Verification items for the finished model (mm, model axes). A direction names the side the tool comes from. Give positions to 0.01 mm unless a question says otherwise; leave off trailing zeros. Order: outer loops, then holes, each group sorted by start corner. A loop starts at its lowest first (then second) coordinate and runs counter-clockwise, first axis right, second up. Notation, with made-up numbers: (32, 63.25) -> (60, 63.25) arc R27 ccw to (60, 88.25) -> close; hole circle Ø1 at (-12.5, 7). An arc over 180 degrees is marked (long way). One line per question, with ' | ' between items. Start each with the question number.
Q1. Mould release check, pull along X, two halves, no side actions. Record for faces 1 (the cylindrical face through (9, 3, 0)), 2 (the flat face through (-130, 0, 0)), 3 (the cylindrical face through (-1.82, -4.76, 3.65)): released by +X, released by -X, zero draft, split by the parting line, or undercut.
Q2. Go/stop test with flat-tipped pins: pin 1 (3.5 mm diameter, centred on x = 7, z = 0, fed in from +Y); pin 2 (3 mm diameter, centred on x = -115, z = 2.5, fed in from +Y); pin 3 (1.5 mm diameter, centred on x = -45, y = -3.5, fed in from -Z). Record where each tip stops, or that it passes through.
Q3. Section check A-A on z = 0. Record the cut outline in (x, y).
Q4. Section check B-B on y = -2.25. Record the cut outline in (x, z).
Q5. Access from +Z, -Z, +X, -X, +Y, -Y to the whole of each face (thin tool, end or side, straight path). Record for faces 4 (the flat face through (7, 0, 0)), 5 (the flat face through (130, 0, 0)), 6 (the flat face through (115, 3, 0)).
Q6. Section check C-C on x = -44. Record the cut outline in (y, z).
Q7. Material ranges on probe 1 along X at (y, z) = (1.5, 0); probe 2 along X at (y, z) = (4.5, 0); probe 3 along X at (y, z) = (4.5, 3.5), recorded low to high. Write a range as [from, to].
Autodesk Inventor part; units mm, degrees
ref_plane "YZ Plane" through (0, 0, 0) normal (1, 0, 0) x (0, 1, 0)
ref_plane "XZ Plane" through (0, 0, 0) normal (0, 1, 0) x (-1, 0, 0)
ref_plane "XY Plane" through (0, 0, 0) normal (0, 0, 1) x (1, 0, 0)
sketch "Sketch1" plane through (0, 0, 0) normal (1, 0, 0) x (0, 1, 0)
  circle A0 centre (0, 0) radius 6
  dimension "d0" = 12
extrude "Extrusion1" add sketch "Sketch1" along normal mid plane 260
sketch "Sketch2" plane through (0, 0, 0) normal (0, 0, 1) x (1, 0, 0)
  line L0 (-130, 6) -> (-130, -6)
  line L1 (-130, 0) -> (-115, 0)
  line L2 (-115, 0) -> (-115, 6)
  line L3 (130, -6) -> (130, 6)
  line L4 (130, 0) -> (115, 0)
  line L5 (115, 0) -> (115, 6)
  line L6 (112, 9) -> (118, 9)
  line L7 (118, 9) -> (118, 3)
  line L8 (118, 3) -> (112, 3)
  line L9 (112, 3) -> (112, 9)
  line L10 (112, 9) -> (118, 3) construction
  line L11 (118, 9) -> (112, 3) construction
  line L12 (-118, 9) -> (-112, 9)
  line L13 (-112, 9) -> (-112, 3)
  line L14 (-112, 3) -> (-118, 3)
  line L15 (-118, 3) -> (-118, 9)
  line L16 (-118, 9) -> (-112, 3) construction
  line L17 (-112, 9) -> (-118, 3) construction
  point P0 (0, 0)
  dimension "d3" = 15
  dimension "d4" = 15
  dimension "d5" = 6
  dimension "d6" = 6
extrude "Extrusion2" cut sketch "Sketch2" along normal mid plane 20
sketch "Sketch3" plane through (0, 0, 0) normal (0, 1, 0) x (-1, 0, 0)
  line L0 (-130, 6) -> (-130, -6)
  line L1 (-130, -6) -> (-5, -6)
  line L2 (130, -6) -> (-130, -6)
  line L3 (-5, -6) -> (-5, 0)
  line L4 (130, 6) -> (-130, 6)
  line L5 (-5, 0) -> (5, 0)
  line L6 (5, 0) -> (7, 0)
  line L7 (-5, 0) -> (-7, 0)
  circle A0 centre (7, 0) radius 2
  circle A1 centre (-7, 0) radius 2
  point P0 (0, 0)
  dimension "d9" = 125
  dimension "d10" = 10
  dimension "d11" = 2
  dimension "d12" = 2
extrude "Extrusion3" cut sketch "Sketch3" along normal blind 10
thread "Thread1"
thread "Thread2"
properties part number "base_axis_12mm" material "Stainless Steel"
Filled in:
1) face 1: undercut | face 2: released by -X | face 3: zero draft
2) pin 1: y = 0 | pin 2: y = 3 | pin 3: z = -5.33
3) outline: (-130, -6) -> (130, -6) -> (130, 6) -> (118, 6) -> (118, 3) -> (112, 3) -> (112, 6) -> (9, 6) -> (9, 0) -> (5, 0) -> (5, 6) -> (-5, 6) -> (-5, 0) -> (-9, 0) -> (-9, 6) -> (-112, 6) -> (-112, 3) -> (-118, 3) -> (-118, 6) -> (-130, 6) -> close
4) outline: (-130, -5.56) -> (130, -5.56) -> (130, 5.56) -> (-130, 5.56) -> close
5) face 4: +Y | face 5: +Z, -Z, +X, +Y, -Y | face 6: +Z, -Z, +Y
6) outline: circle Ø12 at (0, 0)
7) probe 1: [-130, -9], [-5, 5], [9, 130] | probe 2: [-130, -118], [-112, -9], [-5, 5], [9, 112], [118, 130] | probe 3: [-130, -118], [-112, 112], [118, 130]
